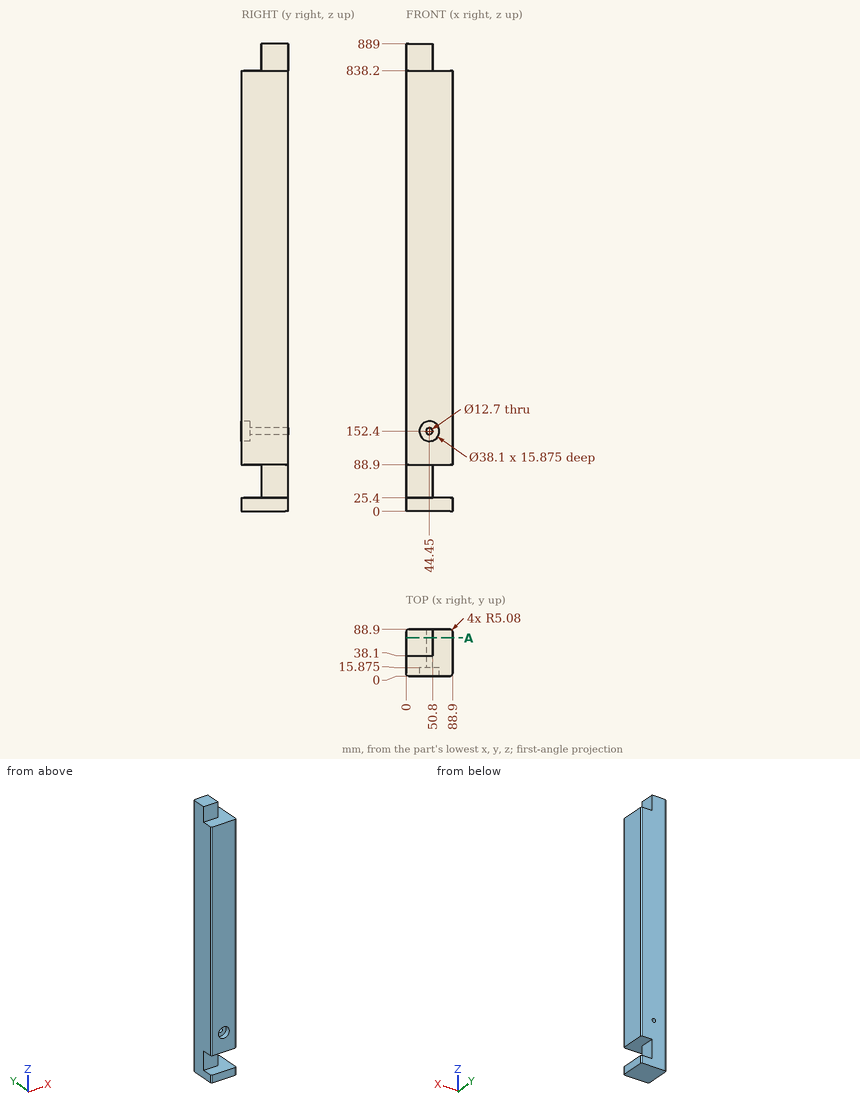
Check sheet for the drawn part. Datum: minimum x, y, z corner. Units: mm. Give positions to 0.01 mm unless a question says otherwise; leave off trailing zeros. Order: outer loops, then holes, each group sorted by start corner. A loop starts at its lowest first (then second) coordinate and runs counter-clockwise, first axis right, second up.
1. Scan lines: line 1 (Z direction, x = 44, y = 5); line 2 (Z direction, x = 44, y = 58); line 3 (X direction, y = 66.5, z = 152.4). Record each from-to range of solid material in increasing order.
Completed:
line 1: z = 0 to 25.4, 88.9 to 133.36, 171.44 to 838.2
line 2: z = 0 to 146.07, 158.73 to 889
line 3: x = 0 to 38.1, 50.8 to 88.9
2. Sectioned sample at A-A (y = 72.5). Record the boundary of the cut face in (x, z).
Completed:
outline: (0, 0) - (88.9, 0) - (88.9, 25.4) - (50.8, 25.4) - (50.8, 88.9) - (88.9, 88.9) - (88.9, 838.2) - (50.8, 838.2) - (50.8, 889) - (0, 889) - close; hole circle Ø12.7 at (44.45, 152.4)
3. Depth check by flat-ended pin: pin 1 (1 mm diameter, centred on x = 57.5, y = 59, fed in from +Z); pin 2 (20.5 mm diameter, centred on x = 44.45, z = 152.4, fed in from -Y) (3 decimals). Enter the tip coordinate at first touch or a pass-through.
Completed:
pin 1: stops at z = 838.2
pin 2: stops at y = 15.875
